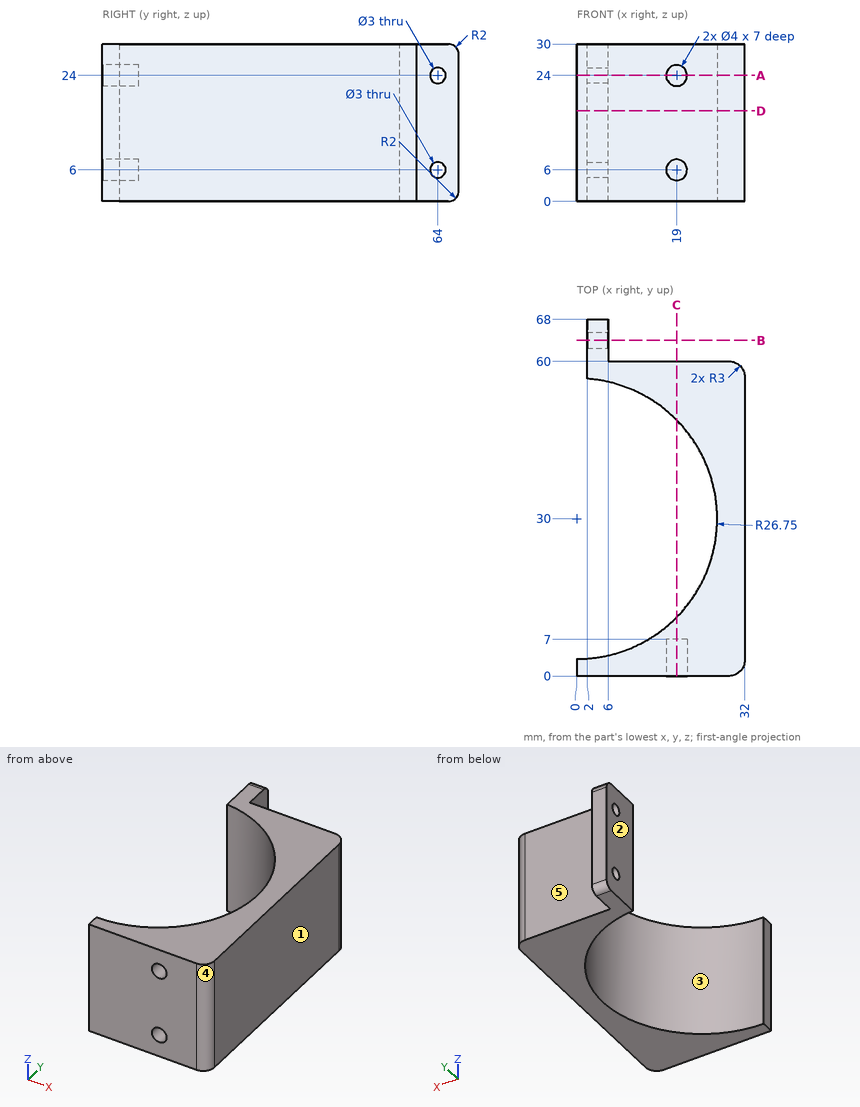
The figure shows three views and two pictorial views of one solid part (mm, origin at its lowest corner). Answer the questions. A direction names the side the tool comes from. Give positions to 0.01 mm unless a question says otherwise; leave off trailing zeros. Write each loop counter-clockwise with the first axis right and the second up, starting at its lowest first coordinate (ties: lowest second). Pieces come first, ordered by that corner, then holes. Notation, with made-up numbers: (25.25, 47.5) - (70.25, 47.5) arc R9 ccw to (70.25, 54.5) - close; hole circle Ø4 at (82, -9.75). An arc over 180 degrees is marked (long way). Return JSON: item names as keys, results as strings.
Q1. For a pull along Y with two mould halves and no side action, classify the marked faces 3, 4 and 5 as released by +Y, released by -Y, zero draft, split by the parting line, or undercut.
Reply:
{"face 3": "undercut", "face 4": "released by -Y", "face 5": "released by +Y"}
Q2. For the marked faces 1 and 2, determine the directions among +Z, -Z, +X, -X, +Y, -Y from which every point of the face is accessible in a straight line to the end or side of a thin tool.
Reply:
{"face 1": "+Z, -Z, +X, +Y, -Y", "face 2": "+Z, -Z, -X, +Y"}
Q3. A cutting plane is placed at B-B, the plane y = 64. Determine the outline of the cut face in (x, z), and give its area (3 significant figures).
Reply:
{"outline": "(2, 0) - (6, 0) - (6, 4.5) - (2, 4.5) - close; (2, 7.5) - (6, 7.5) - (6, 22.5) - (2, 22.5) - close; (2, 25.5) - (6, 25.5) - (6, 30) - (2, 30) - close", "area": "96.0 mm²"}
Q4. A cutting plane is placed at A-A, the plane z = 24. Determine the outline of the cut face in (x, y).
Reply:
{"outline": "(0, 0) - (17, 0) - (17, 7) - (21, 7) - (21, 0) - (29, 0) arc R3 ccw to (32, 3) - (32, 57) arc R3 ccw to (29, 60) - (6, 60) - (6, 62.5) - (2, 62.5) - (2, 56.68) arc R26.75 cw to (0, 3.25) - close; (2, 65.5) - (6, 65.5) - (6, 68) - (2, 68) - close"}
Q5. A cutting plane is placed at D-D, the plane z = 17.25. Determine the outline of the cut face in (x, y), and give its area (3 significant figures).
Reply:
{"outline": "(0, 0) - (29, 0) arc R3 ccw to (32, 3) - (32, 57) arc R3 ccw to (29, 60) - (6, 60) - (6, 68) - (2, 68) - (2, 56.68) arc R26.75 cw to (0, 3.25) - close", "area": "818 mm²"}
Q6. Given P1, Ø3.5, axis at y = 64, z = 24, coming from the -X side; P2, Ø5, axis at x = 13, z = 20, coming from the +Y side; P3, Ø12, axis at y = 45.5, z = 14.5, coming from the -X side, each flat-ended and moving along its own axis, determine where each tip first touches the part or whether it passes through.
Reply:
{"P1": "x = 2", "P2": "y = 60", "P3": "x = 15.92"}
Q7. A cutting plane is placed at C-C, the plane x = 19. Determine the outline of the cut face in (y, z), and give its area (3 significant figures).
Reply:
{"outline": "(0, 0) - (11.17, 0) - (11.17, 30) - (0, 30) - (0, 26) - (7, 26) - (7, 22) - (0, 22) - (0, 8) - (7, 8) - (7, 4) - (0, 4) - close; (48.83, 0) - (60, 0) - (60, 30) - (48.83, 30) - close", "area": "614 mm²"}
Q8. Consider line 1 along Z through (x, y) = (5.15, 64); line 2 along Y through (x, z) = (5.1, 24); line 3 along Y through (x, z) = (4.4, 24). Determine where each line is inside the solid, lowest interval first. Write a range as [from, to].
Reply:
{"line 1": "[0, 4.5], [7.5, 22.5], [25.5, 30]", "line 2": "[0, 3.74], [56.26, 62.5], [65.5, 68]", "line 3": "[0, 3.61], [56.39, 62.5], [65.5, 68]"}
